from build123d import *

# Parameters (mm, degrees)
F0_R       = 3.5
F1_DEPTH   = 3.5
F2_SIZE2   = 1
F2_SIZE    = 0.5
F2_2_SIZE2 = 1
F2_2_SIZE  = 0.5


with BuildPart() as f1:
    # F0 (on Top) → F1 (new body)
    with BuildSketch(Plane.XY):
        with BuildLine():
            ThreePointArc((0, 14), (-7, 7), (0, 0))
            Line((0, 0), (44, 0))
            ThreePointArc((44, 0), (51, 7), (44, 14))
            Line((44, 14), (0, 14))
        make_face()
        with BuildLine():
            ThreePointArc((0, 3.5), (-3.5, 7), (0, 10.5))
            Line((0, 10.5), (11.5, 10.5))
            ThreePointArc((11.5, 10.5), (15, 7), (11.5, 3.5))
            Line((11.5, 3.5), (0, 3.5))
        make_face(mode=Mode.SUBTRACT)
        with Locations((22, 7)):
            Circle(F0_R, mode=Mode.SUBTRACT)
        with BuildLine():
            ThreePointArc((32.5, 3.5), (29, 7), (32.5, 10.5))
            Line((32.5, 10.5), (44, 10.5))
            ThreePointArc((44, 10.5), (47.5, 7), (44, 3.5))
            Line((44, 3.5), (32.5, 3.5))
        make_face(mode=Mode.SUBTRACT)
    extrude(amount=F1_DEPTH)

    # F2
    f2_edges = [f1.edges().sort_by_distance(p)[0] for p in [
        (22, 0, 3.5),
    ]]
    f2_side = f1.faces().sort_by_distance((22, 0.596657, 3.5))[0]
    chamfer(f2_edges, length=F2_SIZE, length2=F2_SIZE2, reference=f2_side)

    # F2#2
    f2_2_edges = [f1.edges().sort_by_distance(p)[0] for p in [
        (22, 0, 0),
    ]]
    f2_2_side = f1.faces().sort_by_distance((22, 0.596657, 0))[0]
    chamfer(f2_2_edges, length=F2_2_SIZE, length2=F2_2_SIZE2, reference=f2_2_side)


solid = f1.part
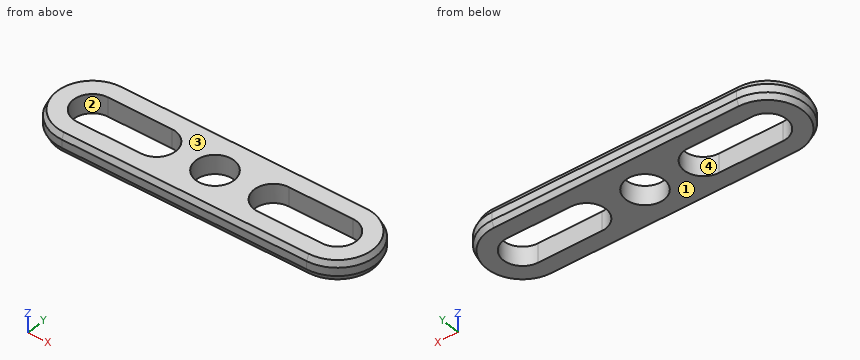
Can you work these out from the model? Positions are in its coordinate system, mm. Face numbers are marked on the shaded views. A direction names the side the tool comes from. Coordinates: 2 decimals unless noted, no trailing zeros. Loops run counter-clockwise (first coordinate to the right, second up) from the corner with the lowest first, then second, coordinate; pieces in that order, holes last. Notation, with made-up numbers: M -34.75,-32 L 7.25,-32 A13 ccw 7.25,-12 Z; hole C -18.5,31.25 d4. An arc over 180 degrees is marked long. Return JSON: item names as keys, results as strings. Group by question number.
Item 1: On a 3-axis mill with a long thin cutter (end or side, diameter ignored), from which of +Z, -Z, +X, -X, +Y, -Y can I reach the whole of each face in a straight line? I mean the marked faces 1 and 2. Say none if no direction works.
Item 2: Imagine slicing it at B-B (y = 7). Please give me the cut outline in (x, z), and give its area (3 significant figures).
Item 3: Imagine slicing it at A-A (x = 22). Please give me the cut outline in (y, z).
Item 4: If I drill on L1, parallel to X at y = 9, z = 0.35; L2, parallel to Y at x = 22, z = 1.1; L3, parallel to X at y = 8.25, z = 1.15, over which ranges is the centre line in solid material (lowest first)? Write a range as from..to.
Item 5: Imagine slicing it at D-D (x = 30). Please give me the cut outline in (y, z), and give its area (3 significant figures).
Item 6: Thinking about a two-plate mould opening in Y: for the marked faces 3 and 4, which applies, released by +Y, released by -Y, zero draft, split by the parting line, or undercut?
Item 7: I'm going to push flat-ended pins straight in: pin 1 Ø1 at (y, z) = (10.5, 2) entering from -X; pin 2 Ø1 at (y, z) = (12.5, 0.5) entering from +X; pin 3 Ø1 at (y, z) = (10.5, 0.5) entering from -X. Where does each tip first touch, or does it pass through?
Item 8: Imagine slicing it at C-C (z = 0.5). Please give me the cut outline in (x, y), and give its area (3 significant figures).
Verdict:
{
 "1": {"face 1": "-Z, +X, -X, +Y, -Y", "face 2": "+Z, -Z"},
 "2": {"outline": "M -7,1 L -6.5,0 L -3.5,0 L -3.5,3.5 L -6.5,3.5 L -7,2.5 Z; M 15,0 L 18.5,0 L 18.5,3.5 L 15,3.5 Z; M 25.5,0 L 29,0 L 29,3.5 L 25.5,3.5 Z; M 47.5,0 L 50.5,0 L 51,1 L 51,2.5 L 50.5,3.5 L 47.5,3.5 Z", "area": "48.0 mm^2"},
 "3": {"outline": "M 0,1 L 0.5,0 L 3.5,0 L 3.5,3.5 L 0.5,3.5 L 0,2.5 Z; M 10.5,0 L 13.5,0 L 14,1 L 14,2.5 L 13.5,3.5 L 10.5,3.5 Z"},
 "4": {"L1": "x = -6.37..-2.87, 14.37..19.13, 24.87..29.63, 46.87..50.37", "L2": "y = 0..3.5, 10.5..14", "L3": "x = -6.89..-3.27, 14.77..18.73, 25.27..29.23, 47.27..50.89"},
 "5": {"outline": "M 0,1 L 0.5,0 L 4.55,0 L 4.55,3.5 L 0.5,3.5 L 0,2.5 Z; M 9.45,0 L 13.5,0 L 14,1 L 14,2.5 L 13.5,3.5 L 9.45,3.5 Z", "area": "30.9 mm^2"},
 "6": {"face 3": "zero draft", "face 4": "undercut"},
 "7": {"pin 1": "stops at x = -6.32", "pin 2": "stops at x = 48.65", "pin 3": "stops at x = -6.17"},
 "8": {"outline": "M 0,0.25 L 44,0.25 A6.75 ccw 44,13.75 L 0,13.75 A6.75 ccw Z; hole M 0,3.5 L 11.5,3.5 A3.5 ccw 11.5,10.5 L 0,10.5 A3.5 ccw Z; hole C 22,7 d7; hole M 32.5,3.5 L 44,3.5 A3.5 ccw 44,10.5 L 32.5,10.5 A3.5 ccw Z", "area": "461 mm^2"}
}
